Here's how the part is built. I have some questions about the finished solid (model axes, mm). A direction names the side the tool comes from. Coordinates: 2 decimals unless noted, no trailing zeros. Order: outer loops, then holes, each group sorted by start corner. A loop starts at its lowest first (then second) coordinate and runs counter-clockwise, first axis right, second up. Notation, with made-up numbers: (22.25, 18.5) - (31.25, 18.5) arc R20 cw to (31.25, 25.5) - close; hole circle Ø2 at (29.25, -14). An arc over 180 degrees is marked (long way). Use CSV: the item, a comma, the result in double quotes. Start each with the question number.
Autodesk Inventor part; units mm, degrees
ref_plane "YZ Plane" through (0, 0, 0) normal (1, 0, 0) x (0, 1, 0)
ref_plane "XZ Plane" through (0, 0, 0) normal (0, 1, 0) x (-1, 0, 0)
ref_plane "XY Plane" through (0, 0, 0) normal (0, 0, 1) x (1, 0, 0)
sketch "Sketch1" plane through (0, 0, 0) normal (0, 1, 0) x (-1, 0, 0)
  line L0 (-12.5, 12.5) -> (12.5, 12.5)
  line L1 (12.5, 12.5) -> (12.5, -12.5)
  line L2 (12.5, -12.5) -> (-12.5, -12.5)
  line L3 (-12.5, -12.5) -> (-12.5, 12.5)
  line L4 (-12.5, 12.5) -> (12.5, -12.5) construction
  line L5 (12.5, 12.5) -> (-12.5, -12.5) construction
  point P0 (0, 0)
  dimension "d0" = 25
  dimension "d1" = 25
extrude "Extrusion1" add sketch "Sketch1" along normal mid plane 3
sketch "Sketch2" plane through (0, 1.5, 0) normal (0, 1, 0) x (1, 0, 0)
  line L0 (12.5, -12.5) -> (12.5, 12.5)
  line L1 (12.5, 12.5) -> (-12.5, 12.5)
  line L2 (12.5, -12.5) -> (9.5, -12.5)
  line L3 (9.5, -12.5) -> (9.5, 12.5)
  line L4 (9.5, 12.5) -> (12.5, 12.5)
  line L5 (12.5, 12.5) -> (12.5, -12.5)
  point P0 (0, 0)
  dimension "d4" = 3
extrude "Extrusion2" add sketch "Sketch2" along normal blind 22
sketch "Sketch3" plane through (12.5, -1.5, 12.5) normal (1, 0, 0) x (0, 0, -1)
  line L0 (25, 0) -> (25, 25)
  line L1 (25, 0) -> (0, 0)
  point P0 (12.5, 1.5)
  point P1 (12.5, 12.5)
  point P2 (25, 12.5)
  point P3 (12.5, 0)
hole "Hole1" at (12.5, 11, 0) direction (-1, 0, 0) diameter 5 end through all
sketch "Sketch4" plane through (0, -1.5, 0) normal (0, -1, 0) x (1, 0, 0)
  point P0 (0, 0)
  point P1 (0, 0)
hole "Hole2" at (0, -1.5, 0) direction (0, 1, 0) diameter 5 end through all
properties part number "WCDLBRACKET"
Item 1: For faces 4 (the flat face through (-4, 1.5, 0)), 5 (the flat face through (-12.5, 0, 0)), which set-ups out of +Z, -Z, +X, -X, +Y, -Y let a thin tool reach every point of the face, with its end or its side?
Item 2: Suppose I cut it at A-A on z = 0. Write out the boundary of the cut face in (x, y).
Item 3: We'd pull the mould along Z, two halves only. Please class faces 1 (the flat face through (9.5, 15, 0)), 2 (the flat face through (10, 5, 12.5)), 3 (the cylindrical face through (2.44, 0.02, 0.54)): released by +Z, released by -Z, zero draft, split by the parting line, or undercut.
Item 4: Suppose I cut it at D-D on y = 0. Write out the boundary of the cut face in (x, z), then the cut area to 3 significant figures.
Item 5: For pin 1 Ø11 at (x, z) = (3.5, -2) entering from +Y; pin 2 Ø11 at (y, z) = (13.5, -0.5) entering from -X, each with a flat end and sliding along its axis, tell me the tip position at first contact or that it passes through.
Item 6: Suppose I cut it at C-C on y = 11. Write out the boundary of the cut face in (x, z).
Item 7: Please list where these lines run through material, in increasing order: line 1 along Z through (x, y) = (0, 0); line 2 along Y through (x, z) = (5.5, -7.5). Write a range as from..to.
Item 8: Suppose I cut it at B-B on x = 0. Write out the boundary of the cut face in (y, z).
Here are the results:
1,face 4,"+Z, -Z, -X, +Y"
1,face 5,"+Z, -Z, -X, +Y, -Y"
2,outline,"(-12.5, -1.5) - (-2.5, -1.5) - (-2.5, 1.5) - (-12.5, 1.5) - close; (2.5, -1.5) - (12.5, -1.5) - (12.5, 8.5) - (9.5, 8.5) - (9.5, 1.5) - (2.5, 1.5) - close; (9.5, 13.5) - (12.5, 13.5) - (12.5, 23.5) - (9.5, 23.5) - close"
3,face 1,"zero draft"
3,face 2,"released by +Z"
3,face 3,"undercut"
4,outline,"(-12.5, -12.5) - (12.5, -12.5) - (12.5, 12.5) - (-12.5, 12.5) - close; hole circle Ø5 at (0, 0)"
4,area,"605 mm^2"
5,pin 1,"y = 1.5"
5,pin 2,"x = 9.5"
6,outline,"(9.5, -12.5) - (12.5, -12.5) - (12.5, -2.5) - (9.5, -2.5) - close; (9.5, 2.5) - (12.5, 2.5) - (12.5, 12.5) - (9.5, 12.5) - close"
7,line 1,"-12.5..-2.5, 2.5..12.5"
7,line 2,"-1.5..1.5"
8,outline,"(-1.5, -12.5) - (1.5, -12.5) - (1.5, -2.5) - (-1.5, -2.5) - close; (-1.5, 2.5) - (1.5, 2.5) - (1.5, 12.5) - (-1.5, 12.5) - close"
